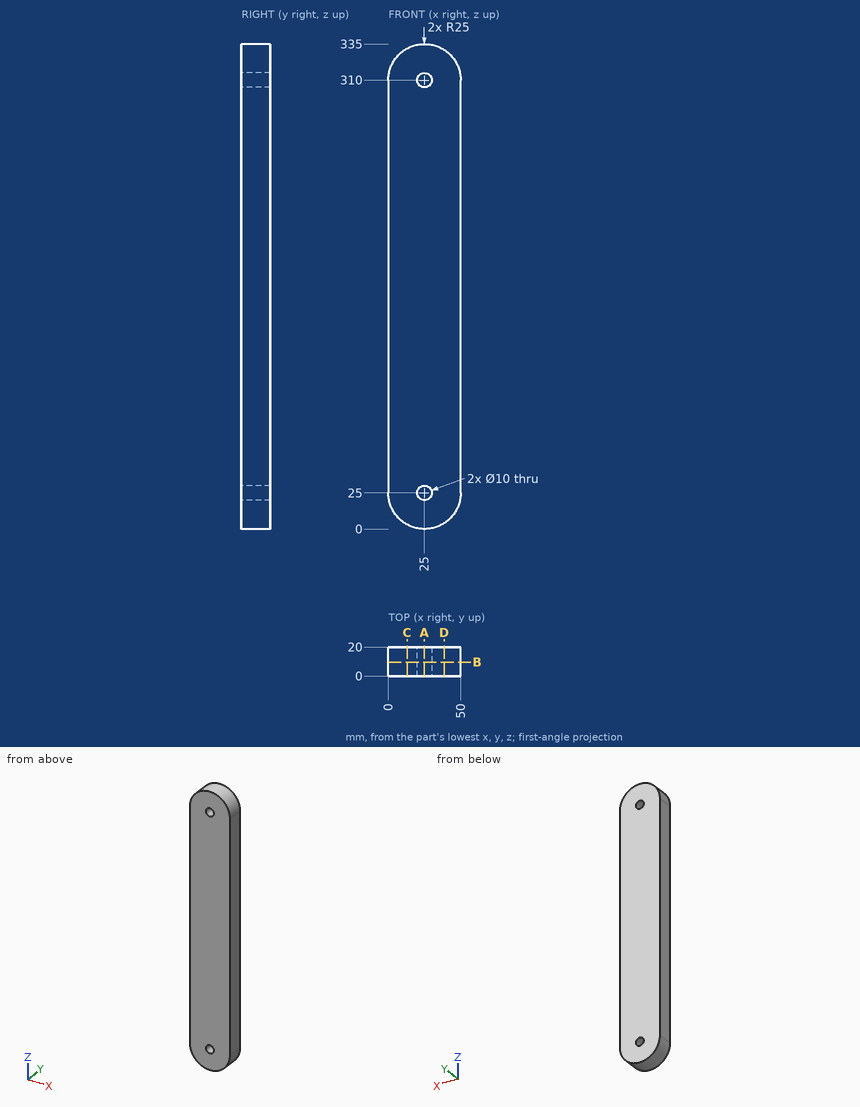
Drawing for the job (mm, zero at the part's lowest x, y, z). Coordinates: 2 decimals unless noted, no trailing zeros. Order: outer loops, then holes, each group sorted by start corner. A loop starts at its lowest first (then second) coordinate and runs counter-clockwise, first axis right, second up. Notation, with made-up numbers: (80.5, 52) -> (118.5, 52) arc R30 cw to (118.5, 75) -> close; hole circle Ø10 at (38, 1). An arc over 180 degrees is marked (long way). One line per item, written item: value.
(1) Probe line 1 (Z direction, x = 25, y = 9.5); line 2 (X direction, y = 10.25, z = 25.5); line 3 (Z direction, x = 24, y = 7). List the from-to ranges inside material, lowest first. Write a range as [from, to].
Checked values:
line 1: [0, 20], [30, 305], [315, 335]
line 2: [0, 20.03], [29.97, 50]
line 3: [0.02, 20.1], [29.9, 305.1], [314.9, 334.98]
(2) Drop flat-ended pins along their axis: pin 1 Ø5 at (x, y) = (10.5, 7) entering from +Z; pin 2 Ø10 at (x, y) = (34, 5.5) entering from -Z; pin 3 Ø8 at (x, z) = (25, 25) entering from +Y; pin 4 Ø3 at (x, y) = (44.5, 11.5) entering from +Z. Give the stop position or say it passes through.
Checked values:
pin 1: z = 331.93
pin 2: z = 0.32
pin 3: through
pin 4: z = 327.35
(3) Slice it at C-C, the plane x = 13. List the corners of the cut face in (y, z), plus the area to 3 significant figures.
Checked values:
outline: (0, 3.07) -> (20, 3.07) -> (20, 331.93) -> (0, 331.93) -> close
area: 6,580 mm2
(4) Slice it at B-B, the plane y = 9.5. List the corners of the cut face in (x, z), plus the area to 3 significant figures.
Checked values:
outline: (0, 25) arc R25 ccw to (50, 25) -> (50, 310) arc R25 ccw to (0, 310) -> close; hole circle Ø10 at (25, 25); hole circle Ø10 at (25, 310)
area: 16,100 mm2
(5) Slice it at D-D, the plane x = 38.5. List the corners of the cut face in (y, z), plus the area to 3 significant figures.
Checked values:
outline: (0, 3.96) -> (20, 3.96) -> (20, 331.04) -> (0, 331.04) -> close
area: 6,540 mm2
(6) Slice it at A-A, the plane x = 25. List the corners of the cut face in (y, z), plus the area to 3 significant figures.
Checked values:
outline: (0, 0) -> (20, 0) -> (20, 20) -> (0, 20) -> close; (0, 30) -> (20, 30) -> (20, 305) -> (0, 305) -> close; (0, 315) -> (20, 315) -> (20, 335) -> (0, 335) -> close
area: 6,300 mm2
